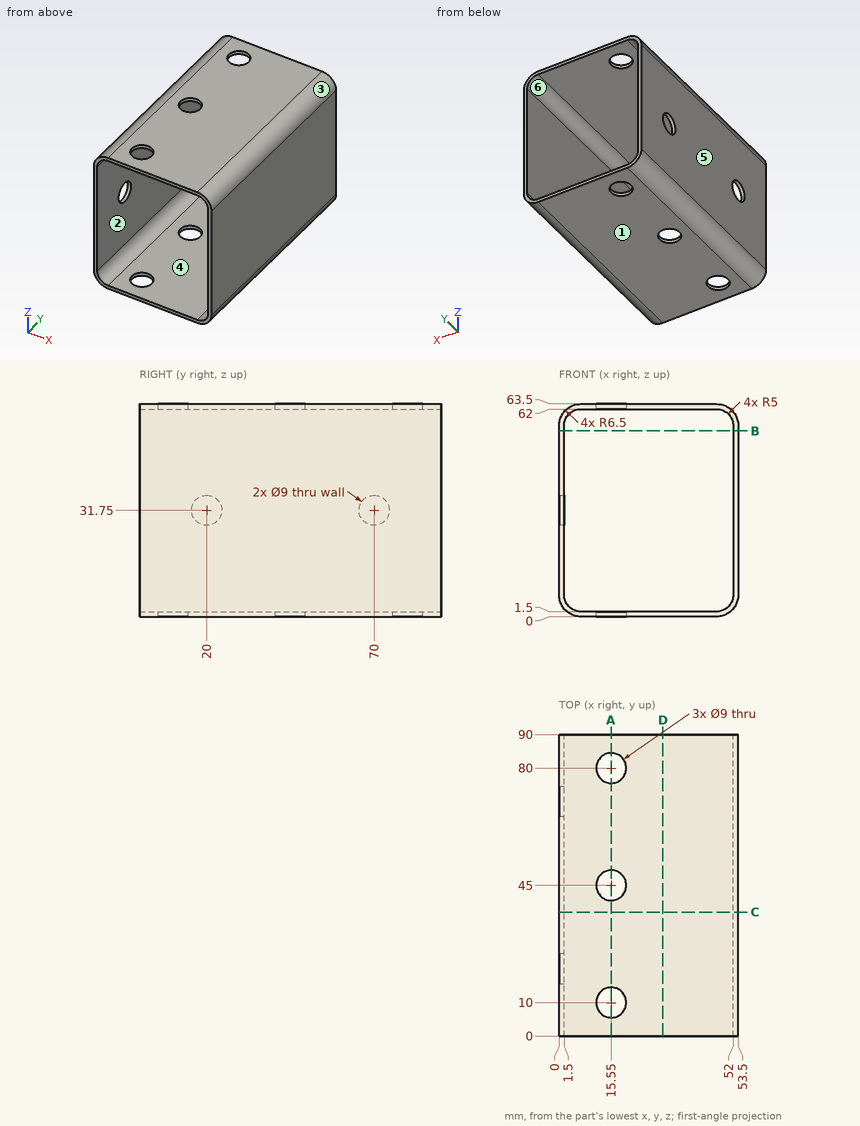
Geometry check sheet. Reference: drawing and pictorial views, mm from the part's lowest x, y, z. A direction names the side the tool comes from. Coordinates: 2 decimals unless noted, no trailing zeros. Order: outer loops, then holes, each group sorted by start corner. A loop starts at its lowest first (then second) coordinate and runs counter-clockwise, first axis right, second up. Notation, with made-up numbers: (-16.75, -25) -> (31.25, -25) arc R19 ccw to (31.25, -6) -> close; hole circle Ø1 at (49.25, 66.5). An arc over 180 degrees is marked (long way). Use CSV: the item, a comma, the result in double quotes. Start each with the question number.
Q1. Depth check by flat-ended pin: P1, Ø14.5, axis at x = 15.55, y = 45, coming from the -Z side; P2, Ø7, axis at y = 20, z = 31.75, coming from the -X side. Enter the tip coordinate at first touch or a pass-through.
Q2. Section check B-B, the plane z = 55.5. Record the cut outline in (x, y), and give its area (3 significant figures).
Q3. Draft check along X on the marked faces 3, 4, 5 and 6. Enter one of: +X half, -X half, draft (parallel to the pull), parting line (faces both ways), or undercut.
Q4. Section check D-D, the plane x = 31. Record the cut outline in (y, z), and give its area (3 significant figures).
Q5. Tool access check on the marked faces 1 and 2. Record the directions out of +Z, -Z, +X, -X, +Y, -Y that give a thin tool (end or side, any length) a straight path to the whole face; none if there is none.
Q6. Section check A-A, the plane x = 15.55. Give the number of separate pieces and of enclosed holes in the cut face, and give its area (3 significant figures).
Q7. Section check C-C, the plane y = 37. Record the cut outline in (x, z).
Q8. Thickness scan on line 1 along Y through (x, z) = (15.55, 1.1); line 2 along Z through (x, y) = (13, 51); line 3 along X through (y, z) = (41, 22). Record the ranges inside material, lowest first.
Returned:
1,P1,"stops at z = 0"
1,P2,"stops at x = 52"
2,outline,"(0, 0) -> (1.5, 0) -> (1.5, 90) -> (0, 90) -> close; (52, 0) -> (53.5, 0) -> (53.5, 90) -> (52, 90) -> close"
2,area,"270 mm^2"
3,face 3,"+X half"
3,face 4,"undercut"
3,face 5,"-X half"
3,face 6,"undercut"
4,outline,"(0, 0) -> (90, 0) -> (90, 1.5) -> (0, 1.5) -> close; (0, 62) -> (90, 62) -> (90, 63.5) -> (0, 63.5) -> close"
4,area,"270 mm^2"
5,face 1,"-Z, +X, -X, +Y, -Y"
5,face 2,"+Y, -Y"
6,separate pieces,"8"
6,enclosed holes,"0"
6,area,"189 mm^2"
7,outline,"(0, 6.5) arc R6.5 ccw to (6.5, 0) -> (47, 0) arc R6.5 ccw to (53.5, 6.5) -> (53.5, 57) arc R6.5 ccw to (47, 63.5) -> (6.5, 63.5) arc R6.5 ccw to (0, 57) -> close; hole (1.5, 6.5) arc R5 ccw to (6.5, 1.5) -> (47, 1.5) arc R5 ccw to (52, 6.5) -> (52, 57) arc R5 ccw to (47, 62) -> (6.5, 62) arc R5 ccw to (1.5, 57) -> close"
8,line 1,"y = 0 to 5.5, 14.5 to 40.5, 49.5 to 75.5, 84.5 to 90"
8,line 2,"z = 0 to 1.5, 62 to 63.5"
8,line 3,"x = 0 to 1.5, 52 to 53.5"
